The model under review builds one solid part; all positions refer to its coordinate system, in mm. Give positions to 0.01 mm unless a question says otherwise; leave off trailing zeros. Loops run counter-clockwise (first coordinate to the right, second up) from the corner with the lowest first, then second, coordinate; pieces in that order, holes last. Notation, with made-up numbers: M 56.5,74 L 105.5,74 A20 cw 105.5,92 Z; hole C 10,55.25 d5. An arc over 180 degrees is marked long. Write item = value, one per line. Start each with the question number.
1. We need section B-B on x = -32.5. Give the boundary of the cut face in (y, z).
2. We need section A-A on y = -30. Give the boundary of the cut face in (x, z).
3. Wall thickness on line 1 along Y through (x, z) = (-32.5, 1.9); line 2 along Y through (x, z) = (-3.5, 0.65): over which ranges is each line inside the solid? List them lowest first. Write a range as from..to.
4. We need section C-C on z = 1.5. Give the boundary of the cut face in (x, y), then the cut area to 3 significant figures.
5. For pin 1 (5.5 mm diameter, centred on x = 88.65, y = -7.75, fed in from +Z), flat-tipped, find the tip position at first contact; note if it passes through.
6. Draft analysis for pull direction X (two halves, no side actions). For faces 1 (the face through (-37.495, -29.78, 1.268)), 2 (the face through (-1, 1, 0)), state which applies: pulls with the +X half, pulls with the -X half, needs draft (parallel to the pull), parting line crosses it, or undercut.
from build123d import *

# Parameters (mm, degrees)
F0_W     = 185
F0_H     = 80
F1_DEPTH = 2.5
F2_R     = 5
F3_DEPTH = 25
F4_R     = 3.5
F5_DEPTH = 25


with BuildPart() as f1:
    # F0 (on Top) → F1 (new body)
    with BuildSketch(Plane.XY):
        Rectangle(F0_W, F0_H)
    extrude(amount=F1_DEPTH)

    # F2 (on face) → F3 (cut)
    with BuildSketch(Plane.XY.offset(2.5)):
        with Locations((-32.5, -30)):
            Circle(F2_R)
        with Locations((0, -30)):
            Circle(F2_R)
        with Locations((-62.919601, -5)):
            Circle(F2_R)
    extrude(amount=-F3_DEPTH, mode=Mode.SUBTRACT)

    # F4 (on face) → F5 (cut)
    with BuildSketch(Plane.XY.offset(2.5)):
        with Locations((88.647544, -7.745902)):
            Circle(F4_R)
    extrude(amount=-F5_DEPTH, mode=Mode.SUBTRACT)


solid = f1.part
Final values:
q1.outline = M -40,0 L -35,0 L -35,2.5 L -40,2.5 Z; M -25,0 L 40,0 L 40,2.5 L -25,2.5 Z
q2.outline = M -92.5,0 L -37.5,0 L -37.5,2.5 L -92.5,2.5 Z; M -27.5,0 L -5,0 L -5,2.5 L -27.5,2.5 Z; M 5,0 L 92.5,0 L 92.5,2.5 L 5,2.5 Z
q3.line_1 = -40..-35, -25..40
q3.line_2 = -40..-33.57, -26.43..40
q4.outline = M -92.5,-40 L 92.5,-40 L 92.5,40 L -92.5,40 Z; hole C -62.92,-5 d10; hole C -32.5,-30 d10; hole C 0,-30 d10; hole C 88.65,-7.75 d7
q4.area = 14,500 mm²
q5.pin_1 = through
q6.face_1 = undercut
q6.face_2 = needs draft
